Read the model definition and answer for the solid it produces. Units are mm, in the model's axes. A direction names the side the tool comes from. Give positions to 0.01 mm unless a question says otherwise; leave off trailing zeros. Write each loop counter-clockwise with the first axis right and the second up, starting at its lowest first coordinate (ties: lowest second). Pieces come first, ordered by that corner, then holes. Notation, with made-up numbers: (26, -7) - (64, -7) arc R25 ccw to (64, 17) - close; hole circle Ø10 at (-8.75, -3.5). An arc over 180 degrees is marked (long way). Answer as CSV lines item,"result".
```python
from build123d import *

# Parameters (mm, degrees)
SKETCH_1_R          = 6
EXTRUDE_1_DEPTH     = 30
SKETCH_2_W          = 22
SKETCH_2_H          = 31
CUT_EXTRUDE_2_DEPTH = 54.935146241
SKETCH_3_R          = 6
CUT_EXTRUDE_3_DEPTH = 30
FILLET_1_R          = 1


with BuildPart() as part:
    # 草图1 → 拉伸1 (new body)
    with BuildSketch(Plane(origin=(0, 0, 0), x_dir=(0, 0, -1), z_dir=(1, 0, 0))):
        with BuildLine():
            Line((0, 0), (0, -21))
            ThreePointArc((0, -21), (14, -35), (28, -21))
            Line((28, -21), (28, 0))
            Line((28, 0), (0, 0))
        make_face()
        with Locations((14, -21)):
            Circle(SKETCH_1_R, mode=Mode.SUBTRACT)
    extrude(amount=EXTRUDE_1_DEPTH)

    # 草图2 → 拉伸2 (cut, through all)
    with BuildSketch(Plane.XY):
        with Locations((15, -19.5)):
            Rectangle(SKETCH_2_W, SKETCH_2_H)
    extrude(amount=-CUT_EXTRUDE_2_DEPTH, mode=Mode.SUBTRACT)

    # 草图3 → 拉伸3 (cut)
    with BuildSketch(Plane(origin=(0, 0, 0), x_dir=(1, 0, 0), z_dir=(0, 1, 0))):
        with Locations(Location((15, 14, 0), (0, 0, 270))):
            Circle(SKETCH_3_R)
    extrude(amount=-CUT_EXTRUDE_3_DEPTH, mode=Mode.SUBTRACT)

    # 圆角1
    fillet_1_edges = [part.edges().sort_by_distance(p)[0] for p in [
        (30, -35, -14),
        (30, -10.5, -28),
        (30, 0, -14),
        (0, -10.5, -28),
        (0, -35, -14),
        (0, -10.5, 0),
        (0, 0, -14),
        (30, -10.5, 0),
        (15, 0, -28),
        (15, 0, 0),
    ]]
    fillet(fillet_1_edges, radius=FILLET_1_R)


solid = part.part
```
(1) Find the intervals of material crossed by L1, parallel to X at y = -1.4, z = -14; L2, parallel to Z at x = 1.2, y = -21; L3, parallel to X at y = -30, z = -19.5, in increasing order.
Worked out:
L1,"x = 0 to 9, 21 to 30"
L2,"z = -28 to -20, -8 to 0"
L3,"x = 0 to 4, 26 to 30"
(2) For faces 5 (the flat face through (26, -13, -14)), 6 (the cylindrical face through (29.699, -10.86, -27.715)), determine the directions among +Z, -Z, +X, -X, +Y, -Y from which every point of the face is accessible in a straight line to the end or side of a thin tool.
Worked out:
face 5,"+Z, -Z, -Y"
face 6,"-Z, +X, +Y, -Y"
(3) A cutting plane is placed at C-C (y = -2.5). Write down the section's boundary in (x, z).
Worked out:
outline,"(0, -27) arc R1 ccw to (1, -28) - (29, -28) arc R1 ccw to (30, -27) - (30, -1) arc R1 ccw to (29, 0) - (1, 0) arc R1 ccw to (0, -1) - close; hole circle Ø12 at (15, -14)"
(4) A cutting plane is placed at A-A (z = -14). Write down the section's boundary in (x, y).
Worked out:
outline,"(0, -34) arc R1 ccw to (1, -35) - (4, -35) - (4, -27) - (0, -27) - close; (0, -15) - (4, -15) - (4, -4) - (9, -4) - (9, 0) - (1, 0) arc R1 ccw to (0, -1) - close; (21, -4) - (26, -4) - (26, -15) - (30, -15) - (30, -1) arc R1 ccw to (29, 0) - (21, 0) - close; (26, -35) - (29, -35) arc R1 ccw to (30, -34) - (30, -27) - (26, -27) - close"
(5) A cutting plane is placed at D-D (x = 2.5). Write down the section's boundary in (y, z).
Worked out:
outline,"(-21, -28) - (-1, -28) arc R1 ccw to (0, -27) - (0, -1) arc R1 ccw to (-1, 0) - (-21, 0) arc R14 ccw to start; hole circle Ø12 at (-21, -14)"
(6) This flat-tipped pin is pushed along its axis until it touches: P1, Ø12, axis at x = 13, z = -16.5, coming from the -Y side. Where does it stop, or does it pass through?
Worked out:
P1,"stops at y = -4"
(7) The mould has two halves that part along X. Classify faces 1 (the cylindrical face through (2, -35, -14)), 2 (the flat face through (30, -14, -14)), 3 (the cylindrical face through (0.285, -0.301, -13.818)), 4 (the flat face through (4, -13, -14)): +X half, -X half, draft (parallel to the pull), parting line (faces both ways), or undercut.
Worked out:
face 1,"draft"
face 2,"+X half"
face 3,"-X half"
face 4,"undercut"
(8) A cutting plane is placed at B-B (x = 15). Write down the section's boundary in (y, z), and give its area (3 significant figures).
Worked out:
outline,"(-4, -28) - (-1, -28) arc R1 ccw to (0, -27) - (0, -20) - (-4, -20) - close; (-4, -8) - (0, -8) - (0, -1) arc R1 ccw to (-1, 0) - (-4, 0) - close"
area,"63.6 mm^2"
